```python
from build123d import *

# Parameters (mm, degrees)
SKETCH1_R               = 28.575
BOSS_EXTRUDE1_DEPTH     = 7.62
SKETCH3_R               = 2.667
SKETCH5_R               = 10.16
BOSS_EXTRUDE3_DEPTH     = 2.54
CUT_EXTRUDE1_DEPTH      = 2.54
CUT_EXTRUDE1_DEPTH_BACK = 2.54
SKETCH6_R               = 1.905
CUT_EXTRUDE2_DEPTH      = 11.16
CUT_EXTRUDE3_DEPTH      = 8.62
SKETCH8_R               = 4.445
CUT_EXTRUDE4_DEPTH      = 1.778


with BuildPart() as part:
    # Sketch1 → Boss-Extrude1 (new body)
    with BuildSketch(Plane.XY):
        Circle(SKETCH1_R)
    extrude(amount=BOSS_EXTRUDE1_DEPTH)

    # Sketch3 → Cut-Revolve1 (revolve, cut)
    with BuildSketch(Plane(origin=(0, 0, 0), x_dir=(0, 0, -1), z_dir=(1, 0, 0))):
        with Locations((-3.81, 29.012456481)):
            Circle(SKETCH3_R)
    revolve(axis=Axis((0, 0, 0), (0, 0, 1)), mode=Mode.SUBTRACT)

    # Sketch5 → Boss-Extrude3 (add)
    with BuildSketch(Plane(origin=(0, 0, 0), x_dir=(-1, 0, 0), z_dir=(0, 0, -1))):
        Circle(SKETCH5_R)
    extrude(amount=BOSS_EXTRUDE3_DEPTH)

    # Sketch4 → Cut-Extrude1 (cut, two sides)
    with BuildSketch(Plane(origin=(0, 0, 0), x_dir=(-1, 0, 0), z_dir=(0, 0, -1))) as cut_extrude1_sk:
        Polygon((7.020938099, 2.976045958), (0.933137647, 7.568333731), (-6.087800452, 4.592287773), (-7.020938099, -2.976045958), (-0.933137647, -7.568333731), (6.087800452, -4.592287773), align=None)
    extrude(amount=CUT_EXTRUDE1_DEPTH, mode=Mode.SUBTRACT)
    extrude(cut_extrude1_sk.sketch, amount=-CUT_EXTRUDE1_DEPTH_BACK, mode=Mode.SUBTRACT)

    # Sketch6 → Cut-Extrude2 (cut, through all)
    with BuildSketch(Plane.XY.offset(7.62)):
        Circle(SKETCH6_R)
    extrude(amount=-CUT_EXTRUDE2_DEPTH, mode=Mode.SUBTRACT)

    # Sketch7 → Cut-Extrude3 (cut, through all)
    with BuildSketch(Plane(origin=(0, 0, 0), x_dir=(-1, 0, 0), z_dir=(0, 0, -1))):
        with BuildLine():
            ThreePointArc((20.358331305, 10.397977999), (12.886311534, 18.881805397), (2.2627084, 22.747741661))
            add(Edge.make_bspline(
                [(2.2627084, 22.747741661), (6.405747391, 20.68512775), (11.177081783, 15.102097432), (11.330348043, 8.533524003), (8.367773099, 5.762462439)],
                knots=[0, 0, 0, 0, 0.593726926, 1, 1, 1, 1], degree=3))
            ThreePointArc((8.367773099, 5.762462439), (9.485052986, 3.641341765), (10.074217449, 1.317475913))
            add(Edge.make_bspline(
                [(20.358331305, 10.397977999), (18.357588554, 2.14920895), (10.074217449, 1.317475913)],
                knots=[0, 0, 0, 1, 1, 1], degree=2))
        make_face()
        with BuildLine():
            ThreePointArc((16.180135083, -16.14877174), (21.939753321, -6.420811804), (22.333603287, 4.877475189))
            add(Edge.make_bspline(
                [(22.333603287, 4.877475189), (21.652210342, 0.299828208), (17.81685639, -5.963231706), (11.617133708, -8.1387974), (8.066211545, -6.17752631)],
                knots=[0, 0, 0, 0, 0.593726926, 1, 1, 1, 1], degree=3))
            ThreePointArc((8.066211545, -6.17752631), (6.394164379, -7.895584962), (4.366098449, -9.174027705))
            add(Edge.make_bspline(
                [(16.180135083, -16.14877174), (7.716826016, -16.794962128), (4.366098449, -9.174027705)],
                knots=[0, 0, 0, 1, 1, 1], degree=2))
        make_face()
        with BuildLine():
            ThreePointArc((-10.358457881, -20.378467811), (0.673201723, -22.850085327), (11.540217523, -19.733296216))
            add(Edge.make_bspline(
                [(11.540217523, -19.733296216), (6.976054533, -20.499823727), (-0.165658961, -18.787577309), (-4.15056456, -13.563577423), (-3.382580204, -9.580383665)],
                knots=[0, 0, 0, 0, 0.593726926, 1, 1, 1, 1], degree=3))
            ThreePointArc((-3.382580204, -9.580383665), (-5.533242071, -8.521081633), (-7.37582021, -6.987336849))
            add(Edge.make_bspline(
                [(-10.358457881, -20.378467811), (-13.588327791, -12.529066385), (-7.37582021, -6.987336849)],
                knots=[0, 0, 0, 1, 1, 1], degree=2))
        make_face()
        with BuildLine():
            ThreePointArc((-22.582014125, 3.554185994), (-21.523691775, -7.701317574), (-15.201356621, -17.07332296))
            add(Edge.make_bspline(
                [(-15.201356621, -17.07332296), (-17.340771534, -12.969416034), (-17.919239259, -5.648129637), (-14.182323678, -0.243954457), (-10.156761081, 0.25652358)],
                knots=[0, 0, 0, 0, 0.593726926, 1, 1, 1, 1], degree=3))
            ThreePointArc((-10.156761081, 0.25652358), (-9.813896046, 2.629266893), (-8.924606034, 4.855616042))
            add(Edge.make_bspline(
                [(-22.582014125, 3.554185994), (-16.114874441, 9.051573254), (-8.924606034, 4.855616042)],
                knots=[0, 0, 0, 1, 1, 1], degree=2))
        make_face()
        with BuildLine():
            ThreePointArc((-3.597994382, 22.575075557), (-13.975574803, 18.090409308), (-20.935172589, 9.181402325))
            add(Edge.make_bspline(
                [(-20.935172589, 9.181402325), (-17.693240732, 12.484283803), (-10.909039954, 15.29684122), (-4.614593512, 13.412805277), (-2.89464336, 9.738923956)],
                knots=[0, 0, 0, 0, 0.593726926, 1, 1, 1, 1], degree=3))
            ThreePointArc((-2.89464336, 9.738923956), (-0.532079248, 10.146057938), (1.860110345, 9.988272599))
            add(Edge.make_bspline(
                [(-3.597994382, 22.575075557), (3.628787662, 18.123246308), (1.860110345, 9.988272599)],
                knots=[0, 0, 0, 1, 1, 1], degree=2))
        make_face()
    extrude(amount=-CUT_EXTRUDE3_DEPTH, mode=Mode.SUBTRACT)

    # Sketch8 → Cut-Extrude4 (cut)
    with BuildSketch(Plane.XY.offset(7.62)):
        Circle(SKETCH8_R)
    extrude(amount=-CUT_EXTRUDE4_DEPTH, mode=Mode.SUBTRACT)


solid = part.part
```
Geometry check sheet. Reference: the model listing, model coordinates, mm. A direction names the side the tool comes from. Coordinates: 2 decimals unless noted, no trailing zeros. Order: outer loops, then holes, each group sorted by start corner. A loop starts at its lowest first (then second) coordinate and runs counter-clockwise, first axis right, second up.
Q1. Sectioned sample at A-A on z = -0.75. Record the cut outline in (x, y), and give its area (3 significant figures).
Reply:
outline: circle Ø20.32 at (0, 0); hole (-7.02, 2.98) - (-6.09, -4.59) - (0.93, -7.57) - (7.02, -2.98) - (6.09, 4.59) - (-0.93, 7.57) - close
area: 173 mm2
Q2. Depth check by flat-ended pin: pin 1 Ø15.5 at (x, y) = (2.5, 1.5) entering from -Z; pin 2 Ø7 at (x, y) = (-0.5, 0.5) entering from +Z; pin 3 Ø1.5 at (x, y) = (-14.5, 16) entering from +Z; pin 4 Ø1 at (y, z) = (-5.5, 4) entering from +X. Enter the tip coordinate at first touch or a pass-through.
Reply:
pin 1: stops at z = -2.54
pin 2: stops at z = 5.84
pin 3: passes through
pin 4: stops at x = 25.9
Q3. Sectioned sample at B-B on y = 19. Give the number of separate pieces and of enclosed holes in the cut face, and give its area (3 significant figures).
Reply:
separate pieces: 3
enclosed holes: 0
area: 160 mm2
Q4. Thickness scan on probe 1 along Y at (x, z) = (12.5, 5); probe 2 along Y at (x, z) = (0, 4.6) (3 decimals); probe 3 along Y at (x, z) = (0, 3.35) (3 decimals). Record the ranges inside material, lowest first.
Reply:
probe 1: y = -23.51 to -0.32, 6.35 to 13.89, 19.14 to 23.51
probe 2: y = -26.465 to -22.86, -17.501 to -1.905, 1.905 to 10.16, 19.484 to 26.465
probe 3: y = -26.385 to -22.86, -17.501 to -1.905, 1.905 to 10.16, 19.484 to 26.385
Q5. Draft check along Y on faces 4 (the face through (0, -12, 0)), 5 (the face through (2.53, 6.1, 0.04)), 6 (the face through (-28.547, 1.256, 0.581)). Enter one of: released by +Y, released by -Y, zero draft, split by the parting line, or undercut.
Reply:
face 4: zero draft
face 5: undercut
face 6: split by the parting line
Q6. Tool access check on faces 1 (the face through (-28.547, 1.256, 7.022)), 2 (the face through (-6.548, -0.861, 0.036)), 3 (the face through (-0.96, -4.34, 6.74)). Record the directions out of +Z, -Z, +X, -X, +Y, -Y that give a thin tool (end or side, any length) a straight path to the whole face; none if there is none.
Reply:
face 1: +Z, -Z
face 2: -Z
face 3: +Z
